Solid Edge part; units mm, degrees
sketch "Sketch1" plane through (0, 0, 0) normal (0, 0, 1) x (1, 0, 0)
  line L0 (17, 9.815) -> (0, 19.6299)
  line L1 (0, 19.6299) -> (-17, 9.815)
  line L2 (-17, 9.815) -> (-17, -9.815)
  line L3 (-17, -9.815) -> (0, -19.6299)
  line L4 (0, -19.6299) -> (17, -9.815)
  line L5 (17, -9.815) -> (17, 9.815)
  circle A0 centre (0, 0) radius 15
extrude "Protrusion1" add sketch "Sketch1" along normal blind 3.85
chamfer "Fase_1" distance 1 angle 45 2 edges at (-15, 0, 3.85) (-15, 0, 0)
sketch "Sketch2" plane through (0, 0, 0) normal (0, -1, 0) x (1, 0, 0)
  line L0 (-24.1454, -0.2754) -> (-9.8546, 7.9754)
  line L1 (-9.8546, 7.9754) -> (-24.1454, 7.9754)
  line L2 (-24.1454, 7.9754) -> (-24.1454, -0.2754)
revolve "RevolvedCutout1" cut sketch "Sketch2" angle 360 about axis through (0, 0, 0) along (0, 0, 1)
mirror "Mirror1" about plane through (-17, 9.815, 1.925) normal (0, 0, 1) of "RevolvedCutout1"
Work out the finished part from the listing and answer in its coordinate system (mm). Round coordinates to 2 decimals unless told otherwise and drop trailing zeros.
Q1. Given pin 1 Ø1 at (x, z) = (-13, 2.5) entering from +Y; pin 2 Ø5 at (x, y) = (13, 8.5) entering from -Z, each flat-ended and moving along its own axis, determine where each tip first touches the part or whether it passes through.
Solution:
pin 1: stops at y = 12.41
pin 2: stops at z = 0
Q2. Find the intervals of material crossed by line 1 along Y through (x, z) = (0, 1.55); line 2 along X through (y, z) = (8.5, 0.2); line 3 along X through (y, z) = (1, 1.65), in increasing order.
Solution:
line 1: y = -19.63 to -15, 15 to 19.63
line 2: x = -15.12 to -13.32, 13.32 to 15.12
line 3: x = -17 to -14.97, 14.97 to 17
Q3. The mould has two halves that part along Y. Classify faces 1 (the conical face through (-0.38, -17.15, 0.09)), 2 (the cylindrical face through (-14.985, -0.66, 1.912)), 3 (the flat face through (17, 0, 2)): pulls with the +Y half, pulls with the -Y half, needs draft (parallel to the pull), parting line crosses it, or undercut.
Solution:
face 1: pulls with the -Y half
face 2: undercut
face 3: needs draft
